Verification items for the finished model (mm, model axes). A direction names the side the tool comes from. Give positions to 0.01 mm unless a question says otherwise; leave off trailing zeros. Loops run counter-clockwise (first coordinate to the right, second up) from the corner with the lowest first, then second, coordinate; pieces in that order, holes last. Notation, with made-up numbers: M -14,20.5 L 28,20.5 A23 ccw 28,34.5 Z; hole C -35,63 d5. An arc over 180 degrees is marked long. Use a Markdown table: item, result.
from build123d import *

# Parameters (mm, degrees)
SKETCH1_W           = 40.894
SKETCH1_H           = 40.132
BOSS_EXTRUDE1_DEPTH = 1.600000102
SKETCH2_R           = 1.90000001
CUT_EXTRUDE1_DEPTH  = 58.318903168
SKETCH2_3_R         = 1.90000001
CUT_EXTRUDE2_DEPTH  = 58.318903168
FILLET1_R           = 2.54
SKETCH5_W           = 40.894
SKETCH5_H           = 46.99
BOSS_EXTRUDE2_DEPTH = 1.600000102
FILLET2_R           = 20.447
SKETCH6_R           = 1.27
CUT_EXTRUDE3_DEPTH  = 75.97959168
CUT_EXTRUDE4_DEPTH  = 75.97959168


with BuildPart() as part:
    # Sketch1 → Boss-Extrude1 (new body)
    with BuildSketch(Plane.XY):
        with Locations((20.447, 20.066)):
            Rectangle(SKETCH1_W, SKETCH1_H)
    extrude(amount=BOSS_EXTRUDE1_DEPTH)

    # Sketch2 → Cut-Extrude1 (cut, through all)
    with BuildSketch(Plane.XY.offset(1.600000102)):
        with Locations((5.200000014, 7.612000016)):
            Circle(SKETCH2_R)
    cut_extrude1 = extrude(amount=-CUT_EXTRUDE1_DEPTH, mode=Mode.SUBTRACT)

    # Sketch2<3> → Cut-Extrude2 (cut, through all)
    with BuildSketch(Plane.XY.offset(1.600000102)):
        with Locations((5.200000014, 31.732000036)):
            Circle(SKETCH2_3_R)
        with Locations((5.200000014, 7.612000016)):
            Circle(SKETCH2_3_R)
    cut_extrude2 = extrude(amount=-CUT_EXTRUDE2_DEPTH, mode=Mode.SUBTRACT)

    # Mirror2: Cut-Extrude1, Cut-Extrude2 across plane
    add(cut_extrude1.mirror(Plane.ZY.offset(-20.447)), mode=Mode.SUBTRACT)
    add(cut_extrude2.mirror(Plane.ZY.offset(-20.447)), mode=Mode.SUBTRACT)

    # Fillet1
    fillet1_edges = [part.edges().sort_by_distance(p)[0] for p in [
        (40.894, 0, 0.800000051),
        (0, 0, 0.800000051),
    ]]
    fillet(fillet1_edges, radius=FILLET1_R)

    # Sketch5 → Boss-Extrude2 (add)
    with BuildSketch(Plane(origin=(0, 40.132, 0), x_dir=(1, 0, 0), z_dir=(0, 1, 0))):
        with Locations((20.447, -23.495)):
            Rectangle(SKETCH5_W, SKETCH5_H)
    extrude(amount=BOSS_EXTRUDE2_DEPTH)

    # Fillet2
    fillet2_edges = [part.edges().sort_by_distance(p)[0] for p in [
        (0, 40.932000051, 46.99),
        (40.894, 40.932000051, 46.99),
    ]]
    fillet(fillet2_edges, radius=FILLET2_R - 0.0001)  # a hair under: the kernel refuses the full size

    # Sketch6 → Cut-Extrude3 (cut, through all)
    with BuildSketch(Plane(origin=(0, 41.732000102, 0), x_dir=(1, 0, 0), z_dir=(0, 1, 0))):
        with Locations(Location((30.226, -39.783999934, 0), (0, 0, 270))):
            Circle(SKETCH6_R)
        with Locations(Location((30.226, -12.954, 0), (0, 0, 270))):
            Circle(SKETCH6_R)
        with Locations(Location((35.480000033, -26.368999967, 0), (0, 0, 270))):
            Circle(SKETCH6_R)
    cut_extrude3 = extrude(amount=-CUT_EXTRUDE3_DEPTH, mode=Mode.SUBTRACT)

    # Mirror3: Cut-Extrude3 across plane
    add(cut_extrude3.mirror(Plane.ZY.offset(-20.447)), mode=Mode.SUBTRACT)

    # Sketch7 → Cut-Extrude4 (cut, through all)
    with BuildSketch(Plane(origin=(0, 41.732000102, 0), x_dir=(1, 0, 0), z_dir=(0, 1, 0))):
        with BuildLine():
            Line((14.605, -34.798), (14.605, -20.066))
            ThreePointArc((14.605, -20.066), (20.447, -14.224), (26.289, -20.066))
            Line((26.289, -20.066), (26.289, -34.798))
            ThreePointArc((26.289, -34.798), (20.447, -40.64), (14.605, -34.798))
        make_face()
    extrude(amount=-CUT_EXTRUDE4_DEPTH, mode=Mode.SUBTRACT)


solid = part.part
(1) Cross-section at C-C on x = 35.48. Record the cut outline in (y, z), then the cut area to 3 significant figures.
Results below:
| item | result |
|---|---|
| outline | M 0,0 L 5.72,0 L 5.72,1.6 L 0,1.6 Z; M 9.5,0 L 29.84,0 L 29.84,1.6 L 9.5,1.6 Z; M 33.62,0 L 41.73,0 L 41.73,25.1 L 40.13,25.1 L 40.13,1.6 L 33.62,1.6 Z; M 40.13,27.64 L 41.73,27.64 L 41.73,40.4 L 40.13,40.4 Z |
| area | 113 mm^2 |
(2) Draft check along Z on faces 4 (the cylindrical face through (11.441, 40.943, 11.946)), 5 (the flat face through (20, 41.732, 13)), 6 (the cylindrical face through (5.83, 40.94, 40.84)), 7 (the cylindrical face through (10.612, 40.943, 38.515)). Enter one of: +Z half, -Z half, draft (parallel to the pull), parting line (faces both ways), or undercut.
Results below:
| item | result |
|---|---|
| face 4 | undercut |
| face 5 | draft |
| face 6 | +Z half |
| face 7 | undercut |
(3) Cross-section at B-B on y = 30.5. Record the cut outline in (x, z), then the cut area to 3 significant figures.
Results below:
| item | result |
|---|---|
| outline | M 0,0 L 3.75,0 L 3.75,1.6 L 0,1.6 Z; M 6.65,0 L 34.25,0 L 34.25,1.6 L 6.65,1.6 Z; M 37.14,0 L 40.89,0 L 40.89,1.6 L 37.14,1.6 Z |
| area | 56.2 mm^2 |
(4) Gauge pin test, flat ends, axial feed: P1, Ø20.5, axis at x = 10.5, z = 20.5, coming from the -Y side; P2, Ø4, axis at x = 12, y = 32, coming from the +Z side; P3, Ø1.3, axis at y = 41, z = 28.5, coming from the +X side. Record the tip position at first contact, or that the pin passes through.
Results below:
| item | result |
|---|---|
| P1 | y = 40.13 |
| P2 | z = 1.6 |
| P3 | x = 40.85 |
(5) Cross-section at A-A on x = 17. Record the cut outline in (y, z).
Results below:
| item | result |
|---|---|
| outline | M 0,0 L 41.73,0 L 41.73,15.35 L 40.13,15.35 L 40.13,1.6 L 0,1.6 Z; M 40.13,39.51 L 41.73,39.51 L 41.73,46.7 L 40.13,46.7 Z |
(6) Cross-section at D-D on z = 9. Record the cut outline in (x, y).
Results below:
| item | result |
|---|---|
| outline | M 0,40.13 L 40.89,40.13 L 40.89,41.73 L 0,41.73 Z |
(7) Set-up check for faces 1 (the flat face through (40.894, 28, 1)), 2 (the flat face through (20, 20, 1.6)), 3 (the flat face through (14.605, 41, 28)): record each of +Z, -Z, +X, -X, +Y, -Y from which the full face is reachable in a straight line by a thin tool's end or side.
Results below:
| item | result |
|---|---|
| face 1 | +Z, -Z, +X, +Y, -Y |
| face 2 | +Z, +X, -X, -Y |
| face 3 | +Y, -Y |
(8) Material ranges on line 1 (Y direction, x = 5.2, z = 1); line 2 (Y direction, x = 26.5, z = 2.5); line 3 (Z direction, x = 14.5, y = 17.5), recorded low to high.
Results below:
| item | result |
|---|---|
| line 1 | 0 to 5.71, 9.51 to 29.83, 33.63 to 41.73 |
| line 2 | 40.13 to 41.73 |
| line 3 | 0 to 1.6 |
